```python
from build123d import *

# Parameters (mm, degrees)
BOX_W             = 19
BOX_H             = 1.8
BOX_DEPTH         = 6
ARRAY004_COUNT    = 6
CYLINDER_R        = 5.75
CYLINDER_DEPTH    = 15
CYLINDER003_R     = 23
CYLINDER003_DEPTH = 17
CYLINDER002_R     = 32.5
CYLINDER002_DEPTH = 17


with BuildPart() as array004:
    # Box → Box (new body)
    with BuildSketch(Plane(origin=(5, -0.9, 0), x_dir=(1, 0, 0), z_dir=(0, 0, 1))):
        with Locations((9.5, 0.9)):
            Rectangle(BOX_W, BOX_H)
    extrude(amount=BOX_DEPTH)

    # Array004: Array004 ×6 about axis
    array004_axis = Axis((0, 0, 0), (0, 0, 1))


with BuildPart() as array004_1:
    add(array004.part)
    for i in range(1, ARRAY004_COUNT):
        add(array004.part.rotate(array004_axis, i * 360 / ARRAY004_COUNT))


with BuildPart() as wheel_model:
    # Cylinder → Cylinder (new body)
    with BuildSketch(Plane.XY):
        Circle(CYLINDER_R)
    extrude(amount=CYLINDER_DEPTH)

    # Fusion: union Array004
    add(array004_1.part)


with BuildPart() as cilindro003:
    # Cylinder003 → Cylinder003 (new body)
    with BuildSketch(Plane.XY):
        Circle(CYLINDER003_R)
    extrude(amount=CYLINDER003_DEPTH)


with BuildPart() as wheel_model001:
    # Cylinder002 → Cylinder002 (new body)
    with BuildSketch(Plane.XY):
        Circle(CYLINDER002_R)
    extrude(amount=CYLINDER002_DEPTH)

    # Cut003: cut Cilindro003
    add(cilindro003.part, mode=Mode.SUBTRACT)

    # Fusion002: union Wheel_model
    add(wheel_model.part)


solid = wheel_model001.part
```
Here's how the part is built. I have some questions about the finished solid (model axes, mm). A direction names the side the tool comes from. Coordinates: 2 decimals unless noted, no trailing zeros. Order: outer loops, then holes, each group sorted by start corner. A loop starts at its lowest first (then second) coordinate and runs counter-clockwise, first axis right, second up.
1) Which directions (+Z, -Z, +X, -X, +Y, -Y) give clear straight access to the entire face, cutting with the end or side of a thin tool? Please do faces 1 (the face through (14, 0, 6)), 2 (the face through (-14, -0.9, 3)).
2) Imagine slicing it at D-D on z = 12.5. List the corners of the cut face in (x, y) for me, and give its area (3 significant figures).
3) Imagine slicing it at A-A on x = 0. List the corners of the cut face in (y, z) for me, and give its area (4 significant figures).
4) Imagine slicing it at B-B on z = 4.5. List the corners of the cut face in (x, y) for me.
5) Imagine slicing it at C-C on y = 0. List the corners of the cut face in (x, z) for me.
6) We'd pull the mould along X, two halves only. Please class faces 3 (the face through (-14, 0.9, 3)), 4 (the face through (6.33, -12.76, 2.96)), 5 (the face through (31, 9.76, 8.38)), 6 (the face through (0, 0, 0)): +X half, -X half, draft (parallel to the pull), parting line (faces both ways), or undercut.
7) Will these pins go through, and if not, where does the flat tip stop? pin 1 (8 mm diameter, centred on x = -7.5, y = -12, fed in from +Z); pin 2 (5 mm diameter, centred on y = 18.5, z = 7.5, fed in from +X); pin 3 (5 mm diameter, centred on x = 5.5, z = 3, fed in from -Y).
8) I need wall thicknesses on line 1 (Y direction, x = 0, z = 7.25); line 2 (X direction, y = -18, z = 2.25); line 3 (X direction, y = 14, z = 5.75). Which ranges of each line are inside material? Lowest first, please.
Response values:
1. face 1: +Z
1. face 2: +Z, -Z
2. outline: circle Ø65 at (0, 0); circle Ø11.5 at (0, 0); hole circle Ø46 at (0, 0)
2. area: 1,760 mm2
3. outline: (-32.5, 0) - (-23, 0) - (-23, 17) - (-32.5, 17) - close; (-5.75, 0) - (5.75, 0) - (5.75, 15) - (-5.75, 15) - close; (23, 0) - (32.5, 0) - (32.5, 17) - (23, 17) - close
3. area: 495.5 mm2
4. outline: circle Ø65 at (0, 0); hole (-22.98, -0.9) arc R23 ccw to (-12.27, -19.45) - (-3.62, -4.47) arc R5.75 cw to (-5.68, -0.9) - close; hole (-22.98, 0.9) - (-5.68, 0.9) arc R5.75 cw to (-3.62, 4.47) - (-12.27, 19.45) arc R23 ccw to start; hole (-10.71, -20.35) arc R23 ccw to (10.71, -20.35) - (2.06, -5.37) arc R5.75 cw to (-2.06, -5.37) - close; hole (-10.71, 20.35) - (-2.06, 5.37) arc R5.75 cw to (2.06, 5.37) - (10.71, 20.35) arc R23 ccw to start; hole (3.62, -4.47) - (12.27, -19.45) arc R23 ccw to (22.98, -0.9) - (5.68, -0.9) arc R5.75 cw to start; hole (3.62, 4.47) arc R5.75 cw to (5.68, 0.9) - (22.98, 0.9) arc R23 ccw to (12.27, 19.45) - close
5. outline: (-32.5, 0) - (32.5, 0) - (32.5, 17) - (23, 17) - (23, 6) - (5.75, 6) - (5.75, 15) - (-5.75, 15) - (-5.75, 6) - (-23, 6) - (-23, 17) - (-32.5, 17) - close
6. face 3: undercut
6. face 4: undercut
6. face 5: parting line
6. face 6: draft
7. pin 1: stops at z = 6
7. pin 2: stops at x = 28.29
7. pin 3: stops at y = -32.36
8. line 1: y = -32.5 to -23, -5.75 to 5.75, 23 to 32.5
8. line 2: x = -27.06 to -14.32, -11.43 to -9.35, 9.35 to 11.43, 14.32 to 27.06
8. line 3: x = -29.33 to -18.25, -9.12 to -7.04, 7.04 to 9.12, 18.25 to 29.33
